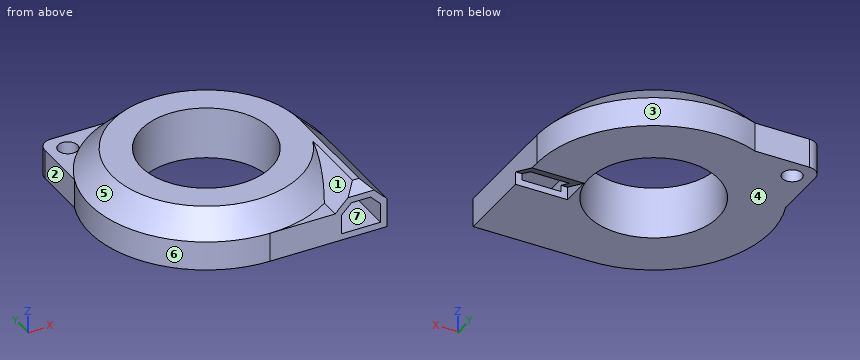
from build123d import *

# Parameters (mm, degrees)
F7_DEPTH       = 18
F8_ANGLE       = 270
F9_DEPTH       = 18
F15_DEPTH      = 6
F16_DEPTH      = 7
F16_DEPTH_BACK = 1
F17_T4_DEPTH   = 22.2867319519
F20_DEPTH      = 4.5
F19_R          = 1.5
F21_DEPTH      = 5
F23_W          = 11.0148127368
F23_H          = 3
F24_DEPTH      = 4.5
F25_SIZE       = 3.5
F26_SIZE       = 1.5


# Not quite as in the source:
# - a fillet or chamfer that OpenCascade refuses, or shapes differently, is made with other operations: its cross-section is extruded or revolved along the edge and cut away or added


with BuildPart() as f5:
    # F0 (on Front) → F5 (revolve)
    with BuildSketch(Plane.XZ):
        Polygon((10, 0), (18, 0), (18, 4.5), (14.5, 8), (10, 8), align=None)
    revolve(axis=Axis((0, 0, 0), (0, 0, 1)))

    # F1 (on Front) → F7 (join)
    with BuildSketch(Plane.XZ):
        Polygon((10, 0), (18, 0), (18, 4.5), (14.5, 8), (10, 8), align=None)
    extrude(amount=F7_DEPTH)


with BuildPart() as f8:
    # F2 (on Front) → F8 (revolve)
    with BuildSketch(Plane.XZ):
        Polygon((10.9985324027, 3.999999641), (11, 1), (17, 1), (17, 4), (14.0656156805, 7), align=None)
    revolve(axis=Axis((0, 0, 0), (0, 0, 1)), revolution_arc=F8_ANGLE)


with BuildPart() as f9:
    # F3 (on Front) → F9 (new body)
    with BuildSketch(Plane.XZ):
        Polygon((11, 4), (11, 1), (17, 1), (17, 4), (14, 7), align=None)
    extrude(amount=F9_DEPTH)


with BuildPart() as f5_1:
    add(f5.part)

    # F10: cut F8
    add(f8.part, mode=Mode.SUBTRACT)

    # F11: cut F9
    add(f9.part, mode=Mode.SUBTRACT)

    # F13 (on offset) → F15 (join)
    with BuildSketch(Plane.YZ.offset(11)):
        Polygon((-6, 7), (-18, 7), (-18, 5.5266313693), (-10, 3), (-6, 3), align=None)
    extrude(amount=F15_DEPTH)

    # F17: chamfer of 2 on 1 edges, made by hand


with BuildPart() as f16:
    # F14 (on offset) → F16 (new body, two sides)
    with BuildSketch(Plane.YZ.offset(11)) as f16_sk:
        Polygon((1, -1), (-6, 2), (-6, -1), align=None)
    extrude(amount=F16_DEPTH)
    extrude(f16_sk.sketch, amount=-F16_DEPTH_BACK)


with BuildPart() as f17_tool2:
    # F17_s3 → F17_t4 (new body)
    with BuildSketch(Plane.XZ.offset(0.8566340241)):
        Polygon((15, 7), (17, 5), (17, 7), align=None)
    extrude(amount=F17_T4_DEPTH)

    split(bisect_by=Plane(origin=(11.25, 0, 11.25), x_dir=(0, 1, 0), z_dir=(0.7071067812, 0, 0.7071067812)), keep=Keep.TOP)


with BuildPart() as f5_2:
    add(f5_1.part)

    # F17_t1: cut F17_tool2
    add(f17_tool2.part, mode=Mode.SUBTRACT)

    # F18: cut F16
    add(f16.part, mode=Mode.SUBTRACT)

    # F6 (on Top) → F20 (join)
    with BuildSketch(Plane.XY):
        with BuildLine():
            Line((-6, 16.8), (-14.8, 16.8))
            ThreePointArc((-14.8, 16.8), (-16.2142135624, 16.2142135624), (-16.8, 14.8))
            Line((-16.8, 14.8), (-16.8, 6))
            Line((-16.8, 6), (-6, 16.8))
        make_face()
    extrude(amount=F20_DEPTH)


with BuildPart() as f21:
    # F19 (on Top) → F21 (new body)
    with BuildSketch(Plane.XY):
        with Locations((-13.8, 13.8)):
            Circle(F19_R)
    extrude(amount=F21_DEPTH)


with BuildPart() as f5_3:
    add(f5_2.part)

    # F22: cut F21
    add(f21.part, mode=Mode.SUBTRACT)

    # F23 (on Top) → F24 (join)
    with BuildSketch(Plane.XY):
        with Locations((5.4925936316, -16.5)):
            Rectangle(F23_W, F23_H)
    extrude(amount=F24_DEPTH)

    # F25
    f25_edges = [f5_3.edges().sort_by_distance(p)[0] for p in [
        (10, -14.25, 8),
    ]]
    chamfer(f25_edges, length=F25_SIZE)

    # F26
    f26_edges = [f5_3.edges().sort_by_distance(p)[0] for p in [
        (14, -18, 8),
    ]]
    chamfer(f26_edges, length=F26_SIZE)


solid = f5_3.part
Can you work these out from the model? Positions are in its coordinate system, mm. Face numbers are marked on the shaded views. A direction names the side the tool comes from. Coordinates: 2 decimals unless noted, no trailing zeros. Write each question's results on one line, items separated by ' | '. Start each with the question number.
Q1. If I drill on probe 1 along Y at (x, z) = (-4, 4.25); probe 2 along Y at (x, z) = (-13.8, 1.3); probe 3 along X at (y, z) = (-12, 1.25), over which ranges is the centre line in solid material (lowest first)?
Q2. I'm going to push flat-ended pins straight in: pin 1 (4 mm diameter, centred on x = -13.5, z = 3.5, fed in from -Y); pin 2 (1 mm diameter, centred on y = 10, z = 5.5, fed in from +X); pin 3 (3 mm diameter, centred on y = -12.5, z = 5.5, fed in from -X). Where does each tip first touch, or does it pass through?
Q3. Imagine slicing it at A-A (y = 8). State how many separate pieces and enclosed holes the cut face has, then the cut area to 3 significant figures.
Q4. We'd pull the mould along Z, two halves only. Please class the marked faces 4, 5, 6 and 7: +Z half, -Z half, draft (parallel to the pull), parting line (faces both ways), or undercut.
Q5. On a 3-axis mill with a long thin cutter (end or side, diameter ignored), from which of +Z, -Z, +X, -X, +Y, -Y can I reach the whole of each face in a straight line? I mean the marked faces 1, 2 and 3. Say none if no direction works.
Taken from the geometry:
1) probe 1: y = -17.55 to -16.27, -10.52 to -9.17, 9.17 to 10.52, 16.27 to 17.55 | probe 2: y = -11.56 to -9.93, 9 to 12.3, 15.3 to 16.8 | probe 3: x = -13.42 to -12.04, 0 to 11, 17 to 18
2) pin 1: stops at y = -13.85 | pin 2: stops at x = 14.45 | pin 3: stops at x = -13.94
3) separate pieces: 2 | enclosed holes: 2 | area: 84.9 mm^2
4) face 4: -Z half | face 5: +Z half | face 6: draft | face 7: undercut
5) face 1: +Z, -Y | face 2: +Z, -Z, -X, +Y | face 3: +Z, -Z, +Y
